```python
from build123d import *

# Parameters (mm, degrees)
SKETCH_W        = 63.5
SKETCH_H        = 44.45
PAD_DEPTH       = 30.48
SKETCH001_W     = 60.96
SKETCH001_H     = 41.91
POCKET_DEPTH    = 29.21
SKETCH002_R     = 2.54
PAD001_DEPTH    = 5.08
SKETCH003_R     = 3.175
POCKET001_DEPTH = 5
COPYSKETCH004_R = 1.016
PAD002_DEPTH    = 3.175


with BuildPart() as part:
    # Sketch → Pad (new body)
    with BuildSketch(Plane.XY):
        with Locations((31.75, 22.225)):
            Rectangle(SKETCH_W, SKETCH_H)
    extrude(amount=PAD_DEPTH)

    # Sketch001 (on Face5 of Pad) → Pocket (cut)
    with BuildSketch(Plane(origin=(0, 0, 0), x_dir=(1, 0, 0), z_dir=(0, 0, -1))):
        with Locations((31.75, -22.225)):
            Rectangle(SKETCH001_W, SKETCH001_H)
    extrude(amount=-POCKET_DEPTH, mode=Mode.SUBTRACT)

    # Sketch002 (on Face11 of Pocket) → Pad001 (join)
    with BuildSketch(Plane(origin=(0, 0, 29.21), x_dir=(1, 0, 0), z_dir=(0, 0, -1))):
        with Locations((3.81, -40.005)):
            Circle(SKETCH002_R)
        with Locations((59.69, -40.005)):
            Circle(SKETCH002_R)
        with Locations((3.81, -3.81)):
            Circle(SKETCH002_R)
        with Locations((59.69, -3.81)):
            Circle(SKETCH002_R)
    extrude(amount=PAD001_DEPTH)

    # Sketch003 (on Face3 of Pad001) → Pocket001 (cut)
    with BuildSketch(Plane.YZ.offset(63.5)):
        with Locations((38.1, 8.89)):
            Circle(SKETCH003_R)
        with BuildLine():
            ThreePointArc((11.43, 11.43), (7.62, 7.62), (11.43, 3.81))
            Line((11.43, 3.81), (14.605, 3.81))
            ThreePointArc((14.605, 3.81), (18.415, 7.62), (14.605, 11.43))
            Line((11.43, 11.43), (14.605, 11.43))
        make_face()
    extrude(amount=-POCKET001_DEPTH, mode=Mode.SUBTRACT)

    # CopySketch004 → Pad002 (join)
    with BuildSketch(Plane(origin=(0, 0, 24.13), x_dir=(1, 0, 0), z_dir=(0, 0, -1))):
        with Locations((3.81, -40.005)):
            Circle(COPYSKETCH004_R)
        with Locations((3.81, -3.81)):
            Circle(COPYSKETCH004_R)
        with Locations((59.69, -3.81)):
            Circle(COPYSKETCH004_R)
        with Locations((59.69, -40.005)):
            Circle(COPYSKETCH004_R)
    extrude(amount=PAD002_DEPTH)


solid = part.part
```
CAD build for the part. Positions are in the model's coordinates, mm. A direction names the side the tool comes from. Give positions to 0.01 mm unless a question says otherwise; leave off trailing zeros. Write each loop counter-clockwise with the first axis right and the second up, starting at its lowest first coordinate (ties: lowest second). Pieces come first, ordered by that corner, then holes. Notation, with made-up numbers: M 36.25,-35.75 L 56.25,-35.75 A32 cw 56.25,-8.75 Z; hole C 35.5,54 d5. An arc over 180 degrees is marked long. Return JSON: item names as keys, results as strings. Group by question number.
(1) Band-saw the part on D-D (z = 8.89). Give the cut face in (x, y) (3 decimals), and give its area (3 significant figures).
(2) Band-saw the part on B-B (z = 15). Give the cut face in (x, y).
(3) 3-axis set-ups, long thin cutter, end or side, ignore diameter. For faces 1 (the face through (1.8, 1.9, 29.21)), 2 (the face through (0, 22, 15)), 3 (the face through (62.874, 35.76, 11.036)): which of +Z, -Z, +X, -X, +Y, -Y reach the whole face in a straight line?
(4) Drill centre lines: L1, parallel to X at y = 22, z = 5.5; L2, parallel to Y at x = 62, z = 8; L3, parallel to Z at x = 63.2, y = 38.1 (3 decimals). Where is each one in solid material? Low to high. Write a range as [from, to].
(5) Flat gauge pins, fed straight in: pin 1 Ø0.6 at (x, y) = (62.5, 12.5) entering from -Z; pin 2 Ø2 at (x, y) = (14, 6.5) entering from -Z; pin 3 Ø1 at (x, y) = (60, 39.5) entering from -Z (3 decimals). Where does each tip first touch, or does it go through?
(6) Mould opens along Z. For faces 4 (the face through (63.5, 22, 15)), 5 (the face through (31, 22, 29.21)), 6 (the face through (62.874, 18.414, 7.536)) say: pulls with the +Z half, pulls with the -Z half, needs draft (parallel to the pull), parting line crosses it, or undercut.
(7) Band-saw the part on A-A (y = 13). Give the cut face in (x, z).
(8) Band-saw the part on C-C (x = 49). Give the cut face in (y, z).
Entries:
{
 "1": {"outline": "M 0,0 L 63.5,0 L 63.5,7.838 L 62.23,7.838 L 62.23,1.27 L 1.27,1.27 L 1.27,43.18 L 62.23,43.18 L 62.23,41.275 L 63.5,41.275 L 63.5,44.45 L 0,44.45 Z; M 62.23,18.197 L 63.5,18.197 L 63.5,34.925 L 62.23,34.925 Z", "area": "247 mm^2"},
 "2": {"outline": "M 0,0 L 63.5,0 L 63.5,44.45 L 0,44.45 Z; hole M 1.27,1.27 L 62.23,1.27 L 62.23,43.18 L 1.27,43.18 Z"},
 "3": {"face 1": "-Z", "face 2": "+Z, -Z, -X, +Y, -Y", "face 3": "+X"},
 "4": {"L1": "x = [0, 1.27], [62.23, 63.5]", "L2": "y = [0, 1.27], [43.18, 44.45]", "L3": "z = [0, 5.715], [12.065, 30.48]"},
 "5": {"pin 1": "stops at z = 0", "pin 2": "stops at z = 29.21", "pin 3": "stops at z = 20.955"},
 "6": {"face 4": "needs draft", "face 5": "pulls with the -Z half", "face 6": "undercut"},
 "7": {"outline": "M 0,0 L 1.27,0 L 1.27,29.21 L 62.23,29.21 L 62.23,11.43 L 63.5,11.43 L 63.5,30.48 L 0,30.48 Z; M 62.23,0 L 63.5,0 L 63.5,3.81 L 62.23,3.81 Z"},
 "8": {"outline": "M 0,0 L 1.27,0 L 1.27,29.21 L 43.18,29.21 L 43.18,0 L 44.45,0 L 44.45,30.48 L 0,30.48 Z"}
}
